Geometry check sheet. Reference: drawing and pictorial views, mm from the part's lowest x, y, z. A direction names the side the tool comes from. Round coordinates to 2 decimals unless told otherwise and drop trailing zeros. Order: outer loops, then holes, each group sorted by start corner. A loop starts at its lowest first (then second) coordinate and runs counter-clockwise, first axis right, second up. Notation, with made-up numbers: (-12, -2) -> (17, -2) arc R22 cw to (17, 37) -> close; hole circle Ø4 at (43, -20.75). An arc over 180 degrees is marked (long way). Return JSON: item names as keys, results as strings. Group by question number.
1) Depth check by flat-ended pin: pin 1 (1.6 mm diameter, centred on y = 26, z = 4.5, fed in from -X); pin 2 (6.5 mm diameter, centred on x = 32, z = 4.5, fed in from +Y); pin 3 (5 mm diameter, centred on x = 3.5, z = 6.5, fed in from -Y). Enter the tip coordinate at first touch or a pass-through.
2) Section check C-C on x = 30. Enter the section's corners in (y, z).
3) Section check A-A on x = 11.75. Enter the section's corners in (y, z) (1 decimal).
4) Section check B-B on z = 10. Enter the section's corners in (x, y).
5) Scan lines: L1, parallel to Z at x = 11.75, y = 26.05 (1 decimal); L2, parallel to X at y = 6.25, z = 11.25; L3, parallel to X at y = 26, z = 3. Record each from-to range of solid material in increasing order.
6) Section check D-D on y = 15.75. Enter the section's corners in (x, z).
7) Tool access check on the marked faces 1, 2 and 3. Record the directions out of +Z, -Z, +X, -X, +Y, -Y that give a thin tool (end or side, any length) a straight path to the whole face; none if there is none.
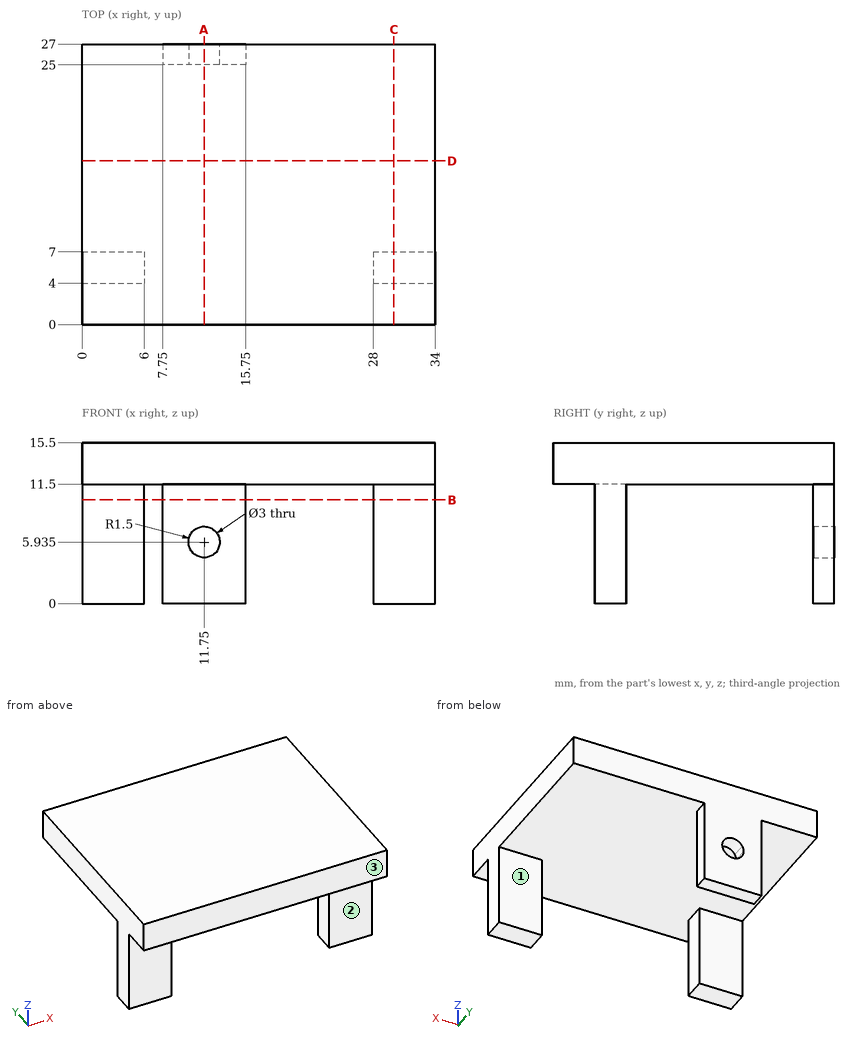
Check result:
{
 "1": {"pin 1": "x = 7.75", "pin 2": "y = 7", "pin 3": "y = 4"},
 "2": {"outline": "(0, 11.5) -> (4, 11.5) -> (4, 0) -> (7, 0) -> (7, 11.5) -> (27, 11.5) -> (27, 15.5) -> (0, 15.5) -> close"},
 "3": {"outline": "(0, 11.5) -> (25, 11.5) -> (25, 7.4) -> (27, 7.4) -> (27, 15.5) -> (0, 15.5) -> close; (25, 0) -> (27, 0) -> (27, 4.4) -> (25, 4.4) -> close"},
 "4": {"outline": "(0, 4) -> (6, 4) -> (6, 7) -> (0, 7) -> close; (7.75, 25) -> (15.75, 25) -> (15.75, 27) -> (7.75, 27) -> close; (28, 4) -> (34, 4) -> (34, 7) -> (28, 7) -> close"},
 "5": {"L1": "0 to 4.4, 7.4 to 15.5", "L2": "0 to 6, 28 to 34", "L3": "7.75 to 15.75"},
 "6": {"outline": "(0, 11.5) -> (34, 11.5) -> (34, 15.5) -> (0, 15.5) -> close"},
 "7": {"face 1": "-Z, +X, -X, +Y", "face 2": "-Z, +X, -X, -Y", "face 3": "+Z, -Z, +X, -X, -Y"}
}
